Input: part model. Units: mm. Frame: model coordinates. A direction names the side the tool comes from. Coordinates: 2 decimals unless noted, no trailing zeros. Order: outer loops, then holes, each group sorted by start corner. A loop starts at its lowest first (then second) coordinate and runs counter-clockwise, first axis right, second up. Notation, with made-up numbers: (-31, 41) -> (-26, 41) arc R36 cw to (-26, 76) -> close; hole circle Ø10 at (76.5, -4). An arc over 180 degrees is marked (long way). One line per question, with ' | ' between items.
```python
from build123d import *

# Parameters (mm, degrees)
F1_DEPTH = 6
F2_DEPTH = 6
F3_R     = 1.25
F4_DEPTH = 21.1718439024
F5_R     = 1.25
F6_DEPTH = 21.1718439024


with BuildPart() as f1:
    # F0 (on Top) → F1 (new body)
    with BuildSketch(Plane.XY):
        Polygon((-6, -18), (6, -18), (6, -10), (18, -10), (18, 18), (6, 18), (6, 10), (-6, 10), (-6, 18), (-18, 18), (-18, -10), (-6, -10), align=None)
        with BuildLine():
            Line((1.5, -12), (1.5, -15))
            ThreePointArc((1.5, -15), (0, -16.5), (-1.5, -15))
            Line((-1.5, -15), (-1.5, -12))
            ThreePointArc((-1.5, -12), (0, -10.5), (1.5, -12))
        make_face(mode=Mode.SUBTRACT)
        with BuildLine():
            ThreePointArc((-13.5, 15), (-12, 16.5), (-10.5, 15))
            Line((-10.5, 15), (-10.5, 12))
            ThreePointArc((-10.5, 12), (-12, 10.5), (-13.5, 12))
            Line((-13.5, 12), (-13.5, 15))
        make_face(mode=Mode.SUBTRACT)
        with BuildLine():
            Line((10.5, 12), (10.5, 15))
            ThreePointArc((10.5, 15), (12, 16.5), (13.5, 15))
            Line((13.5, 15), (13.5, 12))
            ThreePointArc((13.5, 12), (12, 10.5), (10.5, 12))
        make_face(mode=Mode.SUBTRACT)
    extrude(amount=F1_DEPTH)

    # F0 (on Top) → F2 (join)
    with BuildSketch(Plane.XY):
        Polygon((-6, -18), (6, -18), (6, -10), (18, -10), (18, 18), (6, 18), (6, 10), (-6, 10), (-6, 18), (-18, 18), (-18, -10), (-6, -10), align=None)
        with BuildLine():
            Line((1.5, -12), (1.5, -15))
            ThreePointArc((1.5, -15), (0, -16.5), (-1.5, -15))
            Line((-1.5, -15), (-1.5, -12))
            ThreePointArc((-1.5, -12), (0, -10.5), (1.5, -12))
        make_face(mode=Mode.SUBTRACT)
        with BuildLine():
            ThreePointArc((-13.5, 15), (-12, 16.5), (-10.5, 15))
            Line((-10.5, 15), (-10.5, 12))
            ThreePointArc((-10.5, 12), (-12, 10.5), (-13.5, 12))
            Line((-13.5, 12), (-13.5, 15))
        make_face(mode=Mode.SUBTRACT)
        with BuildLine():
            Line((10.5, 12), (10.5, 15))
            ThreePointArc((10.5, 15), (12, 16.5), (13.5, 15))
            Line((13.5, 15), (13.5, 12))
            ThreePointArc((13.5, 12), (12, 10.5), (10.5, 12))
        make_face(mode=Mode.SUBTRACT)
    extrude(amount=F2_DEPTH)

    # F3 (on face) → F4 (cut, through all)
    with BuildSketch(Plane.XZ.offset(10)):
        with Locations((-12, 3)):
            Circle(F3_R)
        with Locations((12, 3)):
            Circle(F3_R)
    extrude(amount=-F4_DEPTH, mode=Mode.SUBTRACT)

    # F5 (on face) → F6 (cut, through all)
    with BuildSketch(Plane(origin=(0, 10, 0), x_dir=(-1, 0, 0), z_dir=(0, 1, 0))):
        with Locations((0, 3)):
            Circle(F5_R)
    extrude(amount=-F6_DEPTH, mode=Mode.SUBTRACT)


solid = f1.part
```
1. Cut plane A-A, the plane y = 2. Return loops of the section in (x, z), and give its area (3 significant figures).
Recorded:
outline: (-18, 0) -> (18, 0) -> (18, 6) -> (-18, 6) -> close; hole circle Ø2.5 at (-12, 3); hole circle Ø2.5 at (0, 3); hole circle Ø2.5 at (12, 3) | area: 201 mm^2
2. Cut plane D-D, the plane x = 7. Return loops of the section in (y, z), and give its area (3 significant figures).
Recorded:
outline: (-10, 0) -> (18, 0) -> (18, 6) -> (-10, 6) -> close | area: 168 mm^2
3. Access query for faces 3 (the face through (0, -16.5, 3)), 4 (the face through (-6, -14, 3)), 5 (the face through (6, 14, 3)), 6 (the face through (0.16, -0.44, 4.24)), 7 (the face through (0, -18, 3)). Directions: +Z, -Z, +X, -X, +Y, -Y. A direction counts if a zero-diameter tool reaches every point of the face in a straight line with its end or side. Return the directions, or none.
Recorded:
face 3: +Z, -Z | face 4: +Z, -Z, -X, -Y | face 5: +Z, -Z, +Y | face 6: +Y | face 7: +Z, -Z, +X, -X, -Y
4. Ray query, line 1 (X direction, y = -4.75, z = 3); line 2 (X direction, y = 14.5, z = 2.25); line 3 (Z direction, x = 12, y = -5). Return the intervals inside material, ascending. Write a range as [from, to].
Recorded:
line 1: x = [-18, -13.25], [-10.75, -1.25], [1.25, 10.75], [13.25, 18] | line 2: x = [-18, -13.5], [-10.5, -6], [6, 10.5], [13.5, 18] | line 3: z = [0, 1.75], [4.25, 6]
5. Cut plane B-B, the plane z = 0.75. Return loops of the section in (x, y), and give its area (3 significant figures).
Recorded:
outline: (-18, -10) -> (-6, -10) -> (-6, -18) -> (6, -18) -> (6, -10) -> (18, -10) -> (18, 18) -> (6, 18) -> (6, 10) -> (-6, 10) -> (-6, 18) -> (-18, 18) -> close; hole (-13.5, 12) arc R1.5 ccw to (-10.5, 12) -> (-10.5, 15) arc R1.5 ccw to (-13.5, 15) -> close; hole (-1.5, -15) arc R1.5 ccw to (1.5, -15) -> (1.5, -12) arc R1.5 ccw to (-1.5, -12) -> close; hole (10.5, 12) arc R1.5 ccw to (13.5, 12) -> (13.5, 15) arc R1.5 ccw to (10.5, 15) -> close | area: 960 mm^2
6. Cut plane C-C, the plane x = 12. Return loops of the section in (y, z), and give its area (4 significant figures).
Recorded:
outline: (-10, 0) -> (10.5, 0) -> (10.5, 1.75) -> (-10, 1.75) -> close; (-10, 4.25) -> (10.5, 4.25) -> (10.5, 6) -> (-10, 6) -> close; (16.5, 0) -> (18, 0) -> (18, 6) -> (16.5, 6) -> close | area: 80.75 mm^2
7. Pin query (flat end, axial travel): pin 1 Ø3 at (y, z) = (-13.5, 3) entering from +X; pin 2 Ø0.9 at (y, z) = (-13, 2.5) entering from -X; pin 3 Ø3 at (x, z) = (1, 0.5) entering from +Y. Return the tip coordinate at first contact, or that it passes through.
Recorded:
pin 1: stops at x = 6 | pin 2: stops at x = -6 | pin 3: stops at y = 10
8. Mould query, pull axis Z, two halves, no side actions, for faces 1 (the face through (-12.921, 0.437, 3.845)), 2 (the face through (-12.1, -10, 1.6)). Classes: released by +Z, released by -Z, zero draft, split by the parting line, or undercut.
Recorded:
face 1: undercut | face 2: zero draft
